Check sheet for the modelled part. Datum: model origin and axes. Units: mm. Face numbers are marked on the shaded views. A direction names the side the tool comes from. Round coordinates to 2 decimals unless told otherwise and drop trailing zeros. Write each loop counter-clockwise with the first axis right and the second up, starting at its lowest first coordinate (ties: lowest second). Pieces come first, ordered by that corner, then holes. Notation, with made-up numbers: (60, 36.5) -> (75, 36.5) arc R17 cw to (75, 46.5) -> close; hole circle Ø1 at (55.5, -35). An arc over 180 degrees is marked (long way). Put each result on its own line as item: value. Start each with the question number.
from build123d import *

# Parameters (mm, degrees)
SKETCH14_R          = 185
SKETCH14_R_2        = 145
SKETCH16_W          = 490
SKETCH16_H          = 490
SKETCH16_R          = 185
BOSS_EXTRUDE1_DEPTH = 50
FILLET2_R           = 20
SKETCH19_R          = 185
BOSS_EXTRUDE2_DEPTH = 50
SKETCH20_R          = 37.5
CUT_EXTRUDE1_DEPTH  = 10
SKETCH26_R          = 17.5
CUT_EXTRUDE3_DEPTH  = 40
CIRPATTERN1_COUNT   = 4
SKETCH28_R          = 37.5
CUT_EXTRUDE4_DEPTH  = 10
SKETCH30_R          = 17.5
CUT_EXTRUDE5_DEPTH  = 40
CIRPATTERN3_COUNT   = 4
CHAMFER1_SIZE       = 10
CHAMFER2_SIZE       = 10


with BuildPart() as part:
    # Sweep-Thin1: sweep along a path in Sketch13
    with BuildLine(Plane.XY) as sweep_thin1_path:
        Line((0, 0), (-150, 0))
        ThreePointArc((-150, 0), (-333.847763109, 76.152236891), (-410, 260))
        Line((-410, 260), (-410, 410))
    # Sketch14 → Sweep-Thin1 (sweep)
    with BuildSketch(Plane(origin=(0, 0, 0), x_dir=(0, 0, -1), z_dir=(1, 0, 0))):
        Circle(SKETCH14_R)
        Circle(SKETCH14_R_2, mode=Mode.SUBTRACT)
    sweep(path=sweep_thin1_path.line)

    # Sketch16 → Boss-Extrude1 (add)
    with BuildSketch(Plane(origin=(0, 0, 0), x_dir=(0, 0, -1), z_dir=(1, 0, 0))):
        Rectangle(SKETCH16_W, SKETCH16_H)
        Circle(SKETCH16_R, mode=Mode.SUBTRACT)
    extrude(amount=-BOSS_EXTRUDE1_DEPTH)

    # Fillet2
    fillet2_edges = [part.edges().sort_by_distance(p)[0] for p in [
        (-25, 245, -245),
        (-25, -245, -245),
        (-25, -245, 245),
        (-25, 245, 245),
    ]]
    fillet(fillet2_edges, radius=FILLET2_R)

    # Sketch19 → Boss-Extrude2 (add)
    with BuildSketch(Plane(origin=(0, 410, 0), x_dir=(1, 0, 0), z_dir=(0, 1, 0))):
        with BuildLine():
            Line((-635, -245), (-185, -245))
            ThreePointArc((-185, -245), (-170.857864376, -239.142135624), (-165, -225))
            Line((-165, -225), (-165, 225))
            ThreePointArc((-165, 225), (-170.857864376, 239.142135624), (-185, 245))
            Line((-185, 245), (-635, 245))
            ThreePointArc((-635, 245), (-649.142135624, 239.142135624), (-655, 225))
            Line((-655, 225), (-655, -225))
            ThreePointArc((-655, -225), (-649.142135624, -239.142135624), (-635, -245))
        make_face()
        with Locations((-410, 0)):
            Circle(SKETCH19_R, mode=Mode.SUBTRACT)
    extrude(amount=-BOSS_EXTRUDE2_DEPTH)

    # Sketch20 → Cut-Extrude1 (cut)
    with BuildSketch(Plane(origin=(0, 410, 0), x_dir=(1, 0, 0), z_dir=(0, 1, 0))):
        with Locations((-605, 195)):
            Circle(SKETCH20_R)
    cut_extrude1 = extrude(amount=-CUT_EXTRUDE1_DEPTH, mode=Mode.SUBTRACT)

    # Sketch26 → Cut-Extrude3 (cut)
    with BuildSketch(Plane(origin=(0, 400, 0), x_dir=(1, 0, 0), z_dir=(0, 1, 0))):
        with Locations((-605, 195)):
            Circle(SKETCH26_R)
    cut_extrude3 = extrude(amount=-CUT_EXTRUDE3_DEPTH, mode=Mode.SUBTRACT)

    # CirPattern1: Cut-Extrude1, Cut-Extrude3 ×4 about axis
    cirpattern1_axis = Axis((-410, 0, 0), (0, 1, 0))
    for i in range(1, CIRPATTERN1_COUNT):
        add(cut_extrude1.rotate(cirpattern1_axis, i * 360 / CIRPATTERN1_COUNT), mode=Mode.SUBTRACT)
        add(cut_extrude3.rotate(cirpattern1_axis, i * 360 / CIRPATTERN1_COUNT), mode=Mode.SUBTRACT)

    # Sketch28 → Cut-Extrude4 (cut)
    with BuildSketch(Plane(origin=(0, 0, 0), x_dir=(0, 0, -1), z_dir=(1, 0, 0))):
        with Locations((-195, 195)):
            Circle(SKETCH28_R)
    cut_extrude4 = extrude(amount=-CUT_EXTRUDE4_DEPTH, mode=Mode.SUBTRACT)

    # Sketch30 → Cut-Extrude5 (cut)
    with BuildSketch(Plane(origin=(-10, 0, 0), x_dir=(0, 0, -1), z_dir=(1, 0, 0))):
        with Locations((-195, 195)):
            Circle(SKETCH30_R)
    cut_extrude5 = extrude(amount=-CUT_EXTRUDE5_DEPTH, mode=Mode.SUBTRACT)

    # CirPattern3: Cut-Extrude4, Cut-Extrude5 ×4 about axis
    cirpattern3_axis = Axis((0, 0, 0), (1, 0, 0))
    for i in range(1, CIRPATTERN3_COUNT):
        add(cut_extrude4.rotate(cirpattern3_axis, i * 360 / CIRPATTERN3_COUNT), mode=Mode.SUBTRACT)
        add(cut_extrude5.rotate(cirpattern3_axis, i * 360 / CIRPATTERN3_COUNT), mode=Mode.SUBTRACT)

    # Chamfer1
    chamfer1_edges = [part.edges().sort_by_distance(p)[0] for p in [
        (0, 0, 145),
    ]]
    chamfer(chamfer1_edges, length=CHAMFER1_SIZE)

    # Chamfer2
    chamfer2_edges = [part.edges().sort_by_distance(p)[0] for p in [
        (-410, 410, 145),
    ]]
    chamfer(chamfer2_edges, length=CHAMFER2_SIZE)


solid = part.part
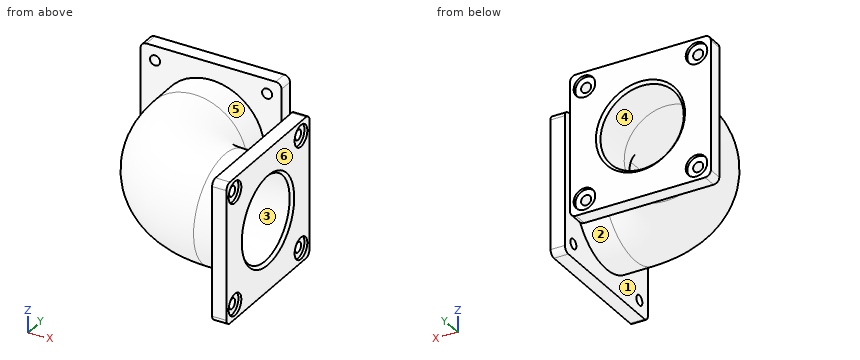
1. Section check B-B, the plane z = 0. Enter the section's corners in (x, y).
2. Access from +Z, -Z, +X, -X, +Y, -Y to the whole of each face (thin tool, end or side, straight path). Record for the marked faces 4, 5 and 6.
3. Section check D-D, the plane z = -195. Give the number of separate pieces and of enclosed holes in the cut face, then the cut area to 3 significant figures.
4. Material ranges on L1, parallel to Z at x = -33, y = -195; L2, parallel to Z at x = -2.75, y = -195, recorded low to high. Write a range as [from, to].
5. Section check C-C, the plane x = -605. Enter the section's corners in (y, z).
6. Section check A-A, the plane y = -195. Enter the section's corners in (x, z).
7. Draft check along Y on the marked faces 1, 2 and 3. Enter one of: released by +Y, released by -Y, zero draft, split by the parting line, or undercut.
8. Gauge pin test, flat ends, axial feed: P1, Ø5, axis at x = -282.5, z = 44.5, coming from the -Y side; P2, Ø12, axis at x = -424, y = 115, coming from the +Z side; P3, Ø3, axis at x = -419, z = 100, coming from the +Y side. Record the tip position at first contact, or that the pin passes through.
Reply:
1. outline: (-655, 360) -> (-595, 360) -> (-595, 260) arc R445 ccw to (-150, -185) -> (-50, -185) -> (-50, -245) -> (0, -245) -> (0, -155) -> (-10, -145) -> (-150, -145) arc R405 cw to (-555, 260) -> (-555, 400) -> (-565, 410) -> (-655, 410) -> close; (-265, 260) arc R115 ccw to (-150, 145) -> (-10, 145) -> (0, 155) -> (0, 245) -> (-50, 245) -> (-50, 185) -> (-150, 185) arc R75 cw to (-225, 260) -> (-225, 360) -> (-165, 360) -> (-165, 410) -> (-255, 410) -> (-265, 400) -> close
2. face 4: +Y
2. face 5: none
2. face 6: +Z, -Z, +X, +Y, -Y
3. separate pieces: 6
3. enclosed holes: 0
3. area: 40,400 mm2
4. L1: z = [-245, -212.5], [-177.5, 177.5], [212.5, 245]
4. L2: z = [-245, -232.5], [-157.5, 157.5], [232.5, 245]
5. outline: (360, -245) -> (410, -245) -> (410, -232.5) -> (400, -232.5) -> (400, -212.5) -> (360, -212.5) -> close; (360, -177.5) -> (400, -177.5) -> (400, -157.5) -> (410, -157.5) -> (410, 157.5) -> (400, 157.5) -> (400, 177.5) -> (360, 177.5) -> close; (360, 212.5) -> (400, 212.5) -> (400, 232.5) -> (410, 232.5) -> (410, 245) -> (360, 245) -> close
6. outline: (-50, -245) -> (0, -245) -> (0, -232.5) -> (-10, -232.5) -> (-10, -212.5) -> (-50, -212.5) -> close; (-50, -177.5) -> (-10, -177.5) -> (-10, -157.5) -> (0, -157.5) -> (0, 157.5) -> (-10, 157.5) -> (-10, 177.5) -> (-50, 177.5) -> close; (-50, 212.5) -> (-10, 212.5) -> (-10, 232.5) -> (0, 232.5) -> (0, 245) -> (-50, 245) -> close
7. face 1: zero draft
7. face 2: split by the parting line
7. face 3: undercut
8. P1: stops at y = -160.13
8. P2: stops at z = 179.69
8. P3: stops at y = 16
